Here's how the part is built. I have some questions about the finished solid (model axes, mm). Face numbers are marked on the shaded views. A direction names the side the tool comes from. Give positions to 0.01 mm unless a question says otherwise; leave off trailing zeros. Loops run counter-clockwise (first coordinate to the right, second up) from the corner with the lowest first, then second, coordinate; pieces in that order, holes last. Notation, with made-up numbers: (18, 83) - (62, 83) arc R19 cw to (62, 110) - close; hole circle Ø10 at (78.5, 62.5). An arc over 180 degrees is marked (long way). Use a Markdown table: item, result.
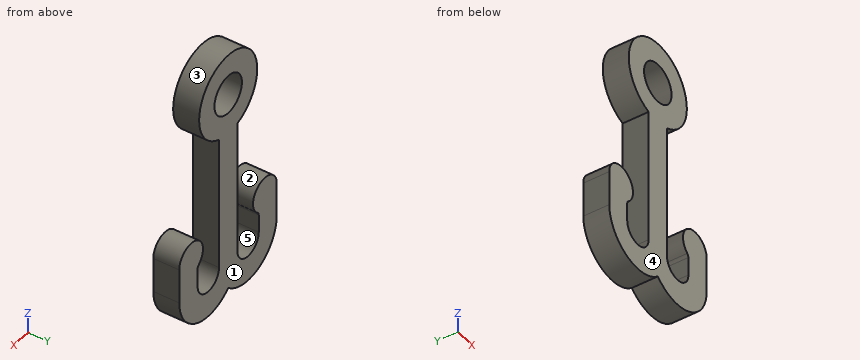
from build123d import *

# Parameters (mm, degrees)
F1_R     = 2.25
F0_DEPTH = 3


with BuildPart() as f0:
    # F1 (on Front) → F0 (new body)
    with BuildSketch(Plane.XZ):
        with BuildLine():
            Line((1.5, -20), (1.5, -4.506939))
            ThreePointArc((1.5, -4.506939), (0, 4.75), (-1.5, -4.506939))
            Line((-1.5, -4.506939), (-1.5, -20))
            ThreePointArc((-1.5, -20), (-3.25, -21.75), (-5, -20))
            Line((-5, -20), (-5, -17.921303))
            ThreePointArc((-5, -17.921303), (-4.949359, -17.702039), (-4.807692, -17.52719))
            ThreePointArc((-4.807692, -17.52719), (-5.15035, -14.258736), (-7.9375, -16))
            Line((-7.9375, -16), (-7.9375, -20))
            ThreePointArc((-7.9375, -20), (-5.087796, -24.296187), (0, -23.464102))
            ThreePointArc((0, -23.464102), (5.137459, -24.358899), (8, -20))
            Line((8, -20), (8, -16))
            ThreePointArc((8, -16), (5.240564, -14.244698), (4.820345, -17.487997))
            ThreePointArc((4.820345, -17.487997), (4.952864, -17.659969), (5, -17.871897))
            Line((5, -17.871897), (5, -20))
            ThreePointArc((5, -20), (3.25, -21.75), (1.5, -20))
        make_face()
        Circle(F1_R, mode=Mode.SUBTRACT)
    extrude(amount=F0_DEPTH)


solid = f0.part
(1) Will these pins go through, and if not, where does the flat tip stop? pin 1 (1 mm diameter, centred on x = -4.5, y = -2, fed in from -Z); pin 2 (1.5 mm diameter, centred on y = -1.5, z = -9, fed in from +X); pin 3 (1 mm diameter, centred on y = -2, z = -0.5, fed in from -X).
A:
| item | result |
|---|---|
| pin 1 | z = -24.62 |
| pin 2 | x = 1.5 |
| pin 3 | x = -4.75 |
(2) If I drill on line 1 (X direction, y = -1.8, z = -15); line 2 (X direction, y = -0.9, z = -10.25); line 3 (Z direction, x = 0.25, y = -1.85), over which ranges is the centre line in solid material (lowest first)?
A:
| item | result |
|---|---|
| line 1 | -7.66 to -4.34, -1.5 to 1.5, 4.4 to 7.72 |
| line 2 | -1.5 to 1.5 |
| line 3 | -23.68 to -2.24, 2.24 to 4.74 |
(3) Suppose I cut it at B-B on x = 3.25. Write out the boundary of the cut face in (y, z).
A:
| item | result |
|---|---|
| outline | (-3, -24.75) - (0, -24.75) - (0, -21.75) - (-3, -21.75) - close; (-3, -3.46) - (0, -3.46) - (0, 3.46) - (-3, 3.46) - close |
(4) Suppose I cut it at A-A on z = 0. Write out the boundary of the cut face in (x, y), plus the area to 3 significant figures.
A:
| item | result |
|---|---|
| outline | (-4.75, -3) - (-2.25, -3) - (-2.25, 0) - (-4.75, 0) - close; (2.25, -3) - (4.75, -3) - (4.75, 0) - (2.25, 0) - close |
| area | 15.0 mm2 |
(5) We'd pull the mould along X, two halves only. Please class the marked faces 1, 2 and 3: pulls with the +X half, pulls with the -X half, needs draft (parallel to the pull), parting line crosses it, or undercut.
A:
| item | result |
|---|---|
| face 1 | needs draft |
| face 2 | undercut |
| face 3 | parting line crosses it |
(6) Suppose I cut it at C-C on z = -15.5. Write out the boundary of the cut face in (x, y).
A:
| item | result |
|---|---|
| outline | (-7.87, -3) - (-4.13, -3) - (-4.13, 0) - (-7.87, 0) - close; (-1.5, -3) - (1.5, -3) - (1.5, 0) - (-1.5, 0) - close; (4.19, -3) - (7.93, -3) - (7.93, 0) - (4.19, 0) - close |
(7) On a 3-axis mill with a long thin cutter (end or side, diameter ignored), from which of +Z, -Z, +X, -X, +Y, -Y can I reach the whole of each face in a straight line? I mean the marked faces 4 and 5. Say none if no direction works.
A:
| item | result |
|---|---|
| face 4 | +Z, -Z, +X, -X, -Y |
| face 5 | +Y, -Y |
